For this review, take the finished solid that the model builds, in its own axes (mm). Face numbers are marked on the shaded views. A direction names the side the tool comes from. Round coordinates to 2 decimals unless told otherwise and drop trailing zeros. Write each loop counter-clockwise with the first axis right and the second up, starting at its lowest first coordinate (ties: lowest second). Pieces come first, ordered by that corner, then holes. Notation, with made-up numbers: (49, -33.5) -> (60, -33.5) arc R25 ccw to (60, 2.5) -> close; hole circle Ø7 at (74.25, 41.25). An arc over 180 degrees is marked (long way). Answer in a Markdown table with one row per item.
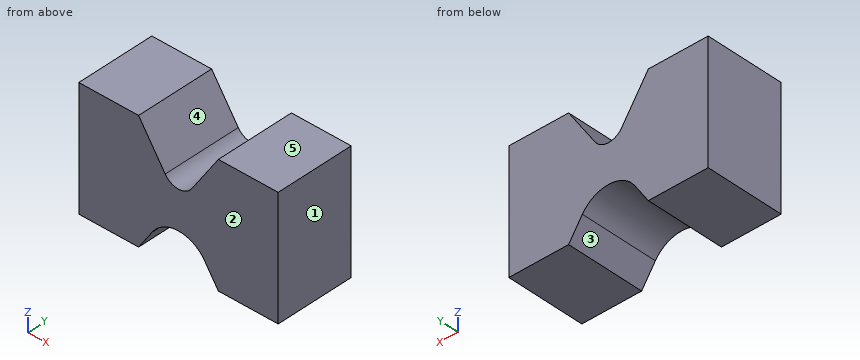
from build123d import *

# Parameters (mm, degrees)
F1_DEPTH = 50
F2_R     = 20


with BuildPart() as f1:
    # F0 (on Front) → F1 (new body)
    with BuildSketch(Plane.XZ):
        with BuildLine():
            Line((-63.5, 38.1), (-63.5, 0))
            Line((-63.5, 0), (-63.5, -38.1))
            Line((-63.5, -38.1), (-25.4, -38.1))
            Line((-25.4, -38.1), (0, 0))
            Line((0, 0), (25.4, -38.1))
            Line((25.4, -38.1), (63.5, -38.1))
            Line((63.5, -38.1), (63.5, 0))
            Line((63.5, 0), (63.5, 38.1))
            Line((63.5, 38.1), (25.4, 38.1))
            Line((25.4, 38.1), (8.453631, 12.680446))
            ThreePointArc((8.453631, 12.680446), (0, 8.1562), (-8.453631, 12.680446))
            Line((-8.453631, 12.680446), (-25.4, 38.1))
            Line((-25.4, 38.1), (-63.5, 38.1))
        make_face()
    extrude(amount=F1_DEPTH)

    # F2
    f2_edges = [f1.edges().sort_by_distance(p)[0] for p in [
        (0, -25, 0),
    ]]
    fillet(f2_edges, radius=F2_R)


solid = f1.part
1) For line 1 (X direction, y = -36.5, z = 16); line 2 (X direction, y = -15, z = -33.5); line 3 (Z direction, x = 11.5, y = -33), list the stretches that pass through material, from the lowest coordinate up. Write a range as [from, to].
Solved:
| item | result |
|---|---|
| line 1 | [-63.5, -10.67], [10.67, 63.5] |
| line 2 | [-63.5, -22.33], [22.33, 63.5] |
| line 3 | [-19.69, 17.25] |
2) Consider section B-B on y = -31. State the section outline as (x, z) points, then the cut area to 3 significant figures.
Solved:
| item | result |
|---|---|
| outline | (-63.5, -38.1) -> (-25.4, -38.1) -> (-16.64, -24.96) arc R20 cw to (16.64, -24.96) -> (25.4, -38.1) -> (63.5, -38.1) -> (63.5, 38.1) -> (25.4, 38.1) -> (8.45, 12.68) arc R10.16 cw to (-8.45, 12.68) -> (-25.4, 38.1) -> (-63.5, 38.1) -> close |
| area | 8,000 mm² |
3) Mouldability with a two-part tool opening along X and no side actions: class the marked faces 1, 2 and 3 as pulls with the +X half, pulls with the -X half, needs draft (parallel to the pull), parting line crosses it, or undercut.
Solved:
| item | result |
|---|---|
| face 1 | pulls with the +X half |
| face 2 | needs draft |
| face 3 | undercut |
4) Consider section A-A on z = 31.5. State the section outline as (x, y) points, then the cut area to 3 significant figures.
Solved:
| item | result |
|---|---|
| outline | (-63.5, -50) -> (-21, -50) -> (-21, 0) -> (-63.5, 0) -> close; (21, -50) -> (63.5, -50) -> (63.5, 0) -> (21, 0) -> close |
| area | 4,250 mm² |
5) For the marked faces 4 and 5, list the 3-axis set-ups (+Z, -Z, +X, -X, +Y, -Y) from which the entire face can be reached by the end or side of a thin tool; tool diameter is ignored.
Solved:
| item | result |
|---|---|
| face 4 | +Z, +Y, -Y |
| face 5 | +Z, +X, -X, +Y, -Y |
6) Consider section C-C on z = -33. State the section outline as (x, y) points.
Solved:
| item | result |
|---|---|
| outline | (-63.5, -50) -> (-22, -50) -> (-22, 0) -> (-63.5, 0) -> close; (22, -50) -> (63.5, -50) -> (63.5, 0) -> (22, 0) -> close |
